Check sheet for the modelled part. Datum: model origin and axes. Units: mm. Face numbers are marked on the shaded views. Round coordinates to 2 decimals unless told otherwise and drop trailing zeros. Order: outer loops, then holes, each group sorted by start corner. A loop starts at its lowest first (then second) coordinate and runs counter-clockwise, first axis right, second up.
Q1. Cross-section at C-C on y = 3.2. Record the cut outline in (x, z) (3 decimals).
Q2. Cross-section at B-B on z = 0. Record the cut outline in (x, y) (3 decimals), then the cut area to 3 significant figures.
Q3. Cross-section at D-D on z = -10. Record the cut outline in (x, y) (3 decimals), then the cut area to 3 significant figures.
Q4. Depth check by flat-ended pin: P1, Ø5, axis at x = 0, z = -10, coming from the -Y side (3 decimals). Enter the tip coordinate at first touch or a pass-through.
Q5. Mould release check, pull along Z, two halves, no side actions. Record for the marked faces 1, 2 and 3: +Z half, -Z half, draft (parallel to the pull), parting line (faces both ways), or undercut.
Q6. Scan lines: probe 1 along Z at (x, y) = (0, 3.8) (3 decimals); probe 2 along X at (y, z) = (1.85, 0) (3 decimals); probe 3 along Z at (x, y) = (-2.75, 2.85). Record each from-to range of solid material in increasing order.
Q7. Cross-section at A-A on x = 0. Record the cut outline in (y, z) (3 decimals).
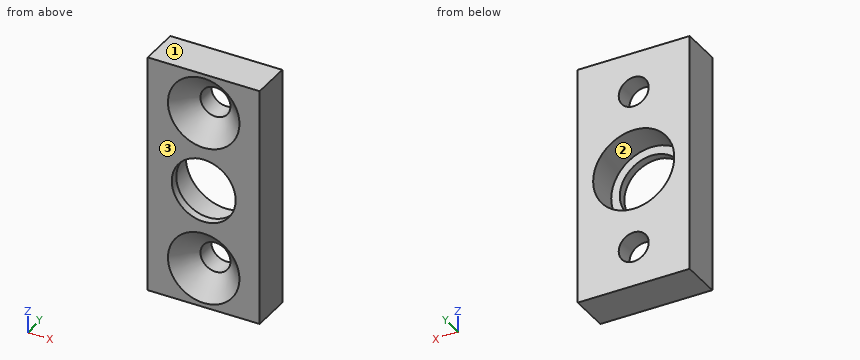
Autodesk Fusion 360 part; units mm, degrees
sketch "Sketch1" plane through (0, 0, 0) normal (0, 1, 0) x (1, 0, 0)
  circle A0 centre (0, 0) radius 5.075
  line L0 (-7, 15) -> (7, 15)
  line L1 (7, 15) -> (7, -15)
  line L2 (7, -15) -> (-7, -15)
  line L3 (-7, -15) -> (-7, 15)
  line L4 (-7, 15) -> (7, -15) construction
  line L5 (7, 15) -> (-7, -15) construction
  dimension "d1" = 10.15
  dimension "d2" = 7
  dimension "d3" = 30
extrude "Extrude1" add sketch "Sketch1" along normal blind 5
sketch "Sketch2" plane through (0, 0, 0) normal (0, -1, 0) x (1, 0, 0)
  circle A0 centre (0, 0) radius 5.075
  line L0 (7, 15) -> (-7, 15)
  line L1 (-7, 15) -> (-7, -15)
  line L2 (-7, -15) -> (7, -15)
  line L3 (7, -15) -> (7, 15)
  line L4 (0, 15) -> (0, -15) construction
  line L5 (0, 0) -> (33.31, 0) construction
  circle A1 centre (0, 10) radius 1.875
  circle A2 centre (0, -10) radius 1.875
  dimension "d6" = 3.75
extrude "Extrude2" cut sketch "Sketch2" against normal blind 31 contours A1 | A2
chamfer "Chamfer1" distance 2.6 angle 45 2 edges at (-1.7481, 0, 10.678) (-1.7481, 0, -9.322)
sketch "Sketch3" plane through (0, 0, 0) normal (0, -1, 0) x (1, 0, 0)
  line L0 (7, -15) -> (7, 15)
  line L1 (7, 15) -> (-7, 15)
  line L2 (-7, 15) -> (-7, -15)
  line L3 (-7, -15) -> (7, -15)
  circle A0 centre (0, 0) radius 5.075
  circle A1 centre (0, 0) radius 4
  circle A2 centre (0, 0) radius 5.075
  circle A3 centre (0, 10) radius 4.475
  circle A4 centre (0, -10) radius 4.475
  dimension "d10" = 8
extrude "Extrude3" add sketch "Sketch3" against normal blind 1 contours A0 A2
Results found:
1. outline: (-7, -15) - (7, -15) - (7, 15) - (-7, 15) - close; hole circle Ø10.15 at (0, 0); hole circle Ø3.75 at (0, -10); hole circle Ø3.75 at (0, 10)
2. outline: (-7, 0) - (-4, 0) - (-4, 1) - (-5.075, 1) - (-5.075, 5) - (-7, 5) - close; (4, 0) - (7, 0) - (7, 5) - (5.075, 5) - (5.075, 1) - (4, 1) - close
2. area: 21.4 mm2
3. outline: (-7, 0) - (-4.475, 0) - (-1.875, 2.6) - (-1.875, 5) - (-7, 5) - close; (1.875, 2.6) - (4.475, 0) - (7, 0) - (7, 5) - (1.875, 5) - close
3. area: 44.5 mm2
4. P1: stops at y = 1.975
5. face 1: +Z half
5. face 2: undercut
5. face 3: draft
6. probe 1: z = -15 to -11.875, -8.125 to -5.075, 5.075 to 8.125, 11.875 to 15
6. probe 2: x = -7 to -5.075, 5.075 to 7
6. probe 3: z = -15 to -4.27, 4.27 to 15
7. outline: (0, -15) - (5, -15) - (5, -11.875) - (2.6, -11.875) - (0, -14.475) - close; (0, -5.525) - (2.6, -8.125) - (5, -8.125) - (5, -5.075) - (1, -5.075) - (1, -4) - (0, -4) - close; (0, 4) - (1, 4) - (1, 5.075) - (5, 5.075) - (5, 8.125) - (2.6, 8.125) - (0, 5.525) - close; (0, 14.475) - (2.6, 11.875) - (5, 11.875) - (5, 15) - (0, 15) - close
